Design review of the part shown in the three views and the two pictorial views. Dimensions are in mm from the part's minimum x, y and z. Round coordinates to 2 decimals unless told otherwise and drop trailing zeros. Order: outer loops, then holes, each group sorted by start corner. A loop starts at its lowest first (then second) coordinate and runs counter-clockwise, first axis right, second up. Notation, with made-up numbers: (-34, 25) - (3, 25) arc R6 cw to (3, 35) - close; hole circle Ø11 at (17, 2). An arc over 180 degrees is marked (long way). One line per question, with ' | ' between items. Start each with the question number.
Item 1: Insertion check: pin 1 Ø2 at (x, y) = (13, 1.5) entering from -Z; pin 2 Ø6 at (x, z) = (3.5, 11.5) entering from -Y; pin 3 Ø1.5 at (y, z) = (1, 16) entering from +X. Each pin has a flat end and moves straight along its axis. Give the tip position at first contact, or say it passes through.
Item 2: For L1, parallel to X at y = 2.25, z = 8.75; L2, parallel to Z at x = 15, y = 2.35; L3, parallel to X at y = 2.35, z = 3.5, list the stretches that pass through material, from the lowest coordinate up. Write a range as [from, to].
Item 3: Add section A-A on y = 2.05. State the section outline as (x, z) points.
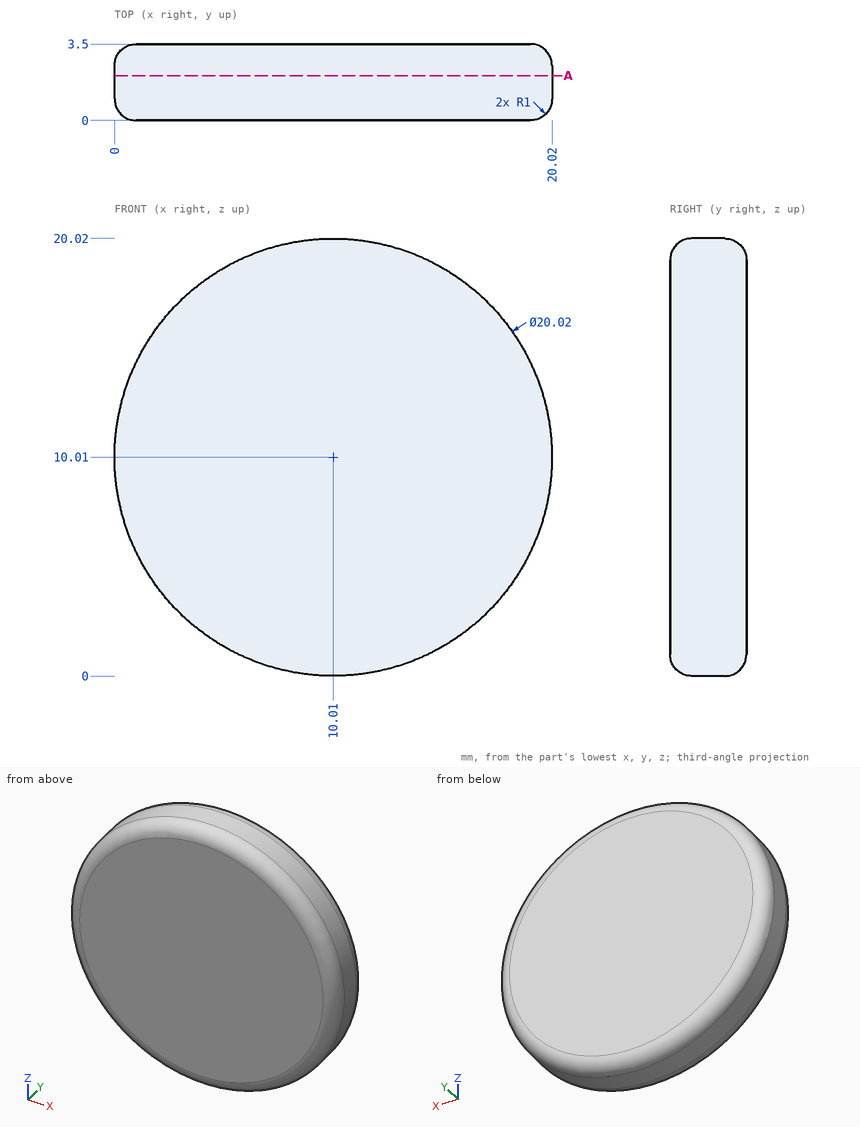
Determined:
1) pin 1: z = 0.2 | pin 2: y = 0 | pin 3: x = 18.54
2) L1: [0.08, 19.94] | L2: [1.33, 18.69] | L3: [2.41, 17.61]
3) outline: circle Ø20.02 at (10.01, 10.01)
